from build123d import *

# Parameters (mm, degrees)
F0_R     = 19.05
F0_R_2   = 4.7625
F1_DEPTH = 19.8374
F0_R_3   = 25.4
F2_DEPTH = 14.859
F4_R     = 1.27


# Not quite as in the source:
# - a fillet or chamfer that OpenCascade refuses, or shapes differently, is made with other operations: its cross-section is extruded or revolved along the edge and cut away or added


with BuildPart() as f1:
    # F0 (on Front) → F1 (new body, symmetric)
    with BuildSketch(Plane.XZ):
        Circle(F0_R)
        Circle(F0_R_2, mode=Mode.SUBTRACT)
    extrude(amount=F1_DEPTH, both=True)

    # F0 (on Front) → F2 (join, symmetric)
    with BuildSketch(Plane.XZ):
        Circle(F0_R_3)
        Circle(F0_R, mode=Mode.SUBTRACT)
    extrude(amount=F2_DEPTH, both=True)

    # F3: chamfer of 6.35 on 2 edges, made by hand


with BuildPart() as f3_tool2:
    # F3_s3 → F3_t4 (revolve)
    with BuildSketch(Plane.XY):
        Polygon((12.7, -19.8374), (19.05, -13.4874), (19.05, -19.8374), align=None)
    revolve(axis=Axis((0, -19.8374, 0), (0, -1, 0)))

    split(bisect_by=Plane.XZ.offset(14.859), keep=Keep.TOP)


with BuildPart() as f1_1:
    add(f1.part)

    # F3_t1: cut F3_tool2
    add(f3_tool2.part, mode=Mode.SUBTRACT)


with BuildPart() as f3_tool7:
    # F3_s8 → F3_t9 (revolve)
    with BuildSketch(Plane.XY):
        Polygon((19.05, 13.4874), (12.7, 19.8374), (19.05, 19.8374), align=None)
    revolve(axis=Axis((0, 19.8374, 0), (0, -1, 0)))

    split(bisect_by=Plane.XZ.offset(-14.859), keep=Keep.BOTTOM)


with BuildPart() as f1_2:
    add(f1_1.part)

    # F3_t6: cut F3_tool7
    add(f3_tool7.part, mode=Mode.SUBTRACT)

    # F4
    f4_edges = [f1_2.edges().sort_by_distance(p)[0] for p in [
        (-25.4, -14.859, 0),
        (-25.4, 14.859, 0),
    ]]
    fillet(f4_edges, radius=F4_R)


solid = f1_2.part
Source: CAD feature listing. Evaluate the final solid. Frame: model axes, mm. A direction names the side the tool comes from. Round coordinates to 2 decimals unless told otherwise and drop trailing zeros. Write each loop counter-clockwise with the first axis right and the second up, starting at its lowest first coordinate (ties: lowest second). Pieces come first, ordered by that corner, then holes. Notation, with made-up numbers: M 72.5,56.25 L 94.5,56.25 A26 cw 94.5,73.25 Z; hole C 53.25,26.25 d3. An arc over 180 degrees is marked long. One line per item, written item: value. Start each with the question number.
Item 1: Set-up query: faces 4 (the conical face through (-12.929, 19.596, 0.569)), 5 (the flat face through (-13, -14.859, 13)). Return all of +Z, -Z, +X, -X, +Y, -Y with unobstructed straight access to the full face (end or side cutting, diameter ignored); none if empty.
Item 2: Section query C-C (y = 9). Return the cut outline in (x, z) (1 decimal).
Item 3: Section query A-A (z = 0). Return the cut outline in (x, y), plus the area to 3 significant figures.
Item 4: Section query B-B (x = 0). Return the cut outline in (y, z).
Item 5: Ray query, L1, parallel to Z at x = 0, y = -5; L2, parallel to Y at x = 3, z = 20.5; L3, parallel to X at y = 8.5, z = 14. Return the intervals inside material, ascending. Write a range as from..to.
Item 6: Pin query (flat end, axial travel): pin 1 (1 mm diameter, centred on x = -19, z = 12, fed in from +Y); pin 2 (6 mm diameter, centred on x = -10, y = -14, fed in from +Z); pin 3 (1.5 mm diameter, centred on x = -7.5, y = -0.5, fed in from +Z). Return the tip coordinate at first contact, or that it passes through.
Item 7: Mould query, pull axis Z, two halves, no side actions, for faces 1 (the cylindrical face through (-3.78, 0.28, -2.9)), 2 (the cylindrical face through (-5.506, -0.19, -24.796)), 3 (the flat face through (-13, 14.859, 13)). Classes: pulls with the +Z half, pulls with the -Z half, needs draft (parallel to the pull), parting line crosses it, or undercut.
Result set:
1. face 4: +Y
1. face 5: -Y
2. outline: C 0,0 d50.8; hole C 0,0 d9.5
3. outline: M -25.4,-13.59 A1.27 ccw -24.13,-14.86 L -17.68,-14.86 L -12.7,-19.84 L -4.76,-19.84 L -4.76,19.84 L -12.7,19.84 L -17.68,14.86 L -24.13,14.86 A1.27 ccw -25.4,13.59 Z; M 4.76,-19.84 L 12.7,-19.84 L 17.68,-14.86 L 24.13,-14.86 A1.27 ccw 25.4,-13.59 L 25.4,13.59 A1.27 ccw 24.13,14.86 L 17.68,14.86 L 12.7,19.84 L 4.76,19.84 Z
3. area: 1,430 mm²
4. outline: M -19.84,-12.7 L -14.86,-17.68 L -14.86,-24.13 A1.27 ccw -13.59,-25.4 L 13.59,-25.4 A1.27 ccw 14.86,-24.13 L 14.86,-17.68 L 19.84,-12.7 L 19.84,-4.76 L -19.84,-4.76 Z; M -19.84,4.76 L 19.84,4.76 L 19.84,12.7 L 14.86,17.68 L 14.86,24.13 A1.27 ccw 13.59,25.4 L -13.59,25.4 A1.27 ccw -14.86,24.13 L -14.86,17.68 L -19.84,12.7 Z
5. L1: z = -25.4..-4.76, 4.76..25.4
5. L2: y = -14.86..14.86
5. L3: x = -21.19..21.19
6. pin 1: stops at y = 14.86
6. pin 2: stops at z = 24.41
6. pin 3: stops at z = 24.49
7. face 1: undercut
7. face 2: parting line crosses it
7. face 3: needs draft
